from build123d import *

# Parameters (mm, degrees)
SKETCH1_W                        = 92.075
SKETCH1_H                        = 15.875
BOSS_EXTRUDE1_DEPTH              = 15.875
SKETCH2_W                        = 47.625
SKETCH2_H                        = 15.875
CUT_EXTRUDE1_DEPTH               = 52.219943931
F_10_0_1935_DIAMETER_HOLE1_D     = 5.1054
F_10_START                       = -7.9375
F_10_0_1935_DIAMETER_SLOT1_DEPTH = 15.875
CUT_EXTRUDE2_REACH               = 51.34
SKETCH7_W                        = 47.625
SKETCH7_H                        = 12.065
CUT_EXTRUDE3_REACH               = 58.485
SKETCH8_W                        = 38.1
SKETCH8_H                        = 9.525
SKETCH9_W                        = 18.415
SKETCH9_H                        = 15.875
BOSS_EXTRUDE2_DEPTH              = 3.81


# Read off the part's stored shape, not the designer's step: #10 (0.1935) Diameter Slot1
with BuildPart() as part:
    # Sketch1 → Boss-Extrude1 (new, symmetric)
    with BuildSketch(Plane(origin=(0, 0, 0), x_dir=(1, 0, 0), z_dir=(0, 1, 0))):
        Rectangle(SKETCH1_W, SKETCH1_H)
    extrude(amount=BOSS_EXTRUDE1_DEPTH, both=True)

    # Sketch2 → Cut-Extrude1 (cut, through all)
    with BuildSketch(Plane.XY.offset(7.9375)):
        with Locations((-22.225, 7.9375)):
            Rectangle(SKETCH2_W, SKETCH2_H)
    extrude(amount=-CUT_EXTRUDE1_DEPTH, mode=Mode.SUBTRACT)

    # #10 (0.1935) Diameter Hole1 (through all)
    with Locations(Plane.XY.offset(7.9375)):
        with Locations((33.3375, 9.525), (20.6375, 9.525)):
            Hole(F_10_0_1935_DIAMETER_HOLE1_D / 2)

    # #10 (0.1935) Diameter Slot1 outline → #10 (0.1935) Diameter Slot1 (cut)
    with BuildSketch(Plane.XY.offset(F_10_START)):
        with BuildLine():
            ThreePointArc((-23.1902, -10.4902), (-20.6375, -7.9375), (-23.1902, -5.3848))
            Line((-23.1902, -5.3848), (-46.0375, -5.3848))
            Line((-46.0375, -5.3848), (-46.0375, -10.4902))
            Line((-46.0375, -10.4902), (-23.1902, -10.4902))
        make_face()
    extrude(amount=F_10_0_1935_DIAMETER_SLOT1_DEPTH, mode=Mode.SUBTRACT)

    # Sketch7 → Cut-Extrude2 (cut, up to next)
    with BuildSketch(Plane(origin=(0, 0, 0), x_dir=(1, 0, 0), z_dir=(0, 1, 0)), mode=Mode.PRIVATE) as cut_extrude2_sk1:
        with Locations((-22.225, 1.905)):
            Rectangle(SKETCH7_W, SKETCH7_H)
    cut_extrude2_tool1 = extrude(cut_extrude2_sk1.sketch, amount=-CUT_EXTRUDE2_REACH, mode=Mode.PRIVATE) & part.part
    add(cut_extrude2_tool1.solids().sort_by_distance((-22.225, 0, -1.905))[0], mode=Mode.SUBTRACT)

    # Sketch8 → Cut-Extrude3 (cut, up to next)
    with BuildSketch(Plane(origin=(0, 15.875, 0), x_dir=(1, 0, 0), z_dir=(0, 1, 0)), mode=Mode.PRIVATE) as cut_extrude3_sk1:
        with Locations((26.9875, -3.175)):
            Rectangle(SKETCH8_W, SKETCH8_H)
    cut_extrude3_tool1 = extrude(cut_extrude3_sk1.sketch, amount=-CUT_EXTRUDE3_REACH, mode=Mode.PRIVATE) & part.part
    add(cut_extrude3_tool1.solids().sort_by_distance((26.9875, 15.875, 3.175))[0], mode=Mode.SUBTRACT)

    # Sketch9 → Boss-Extrude2 (add)
    with BuildSketch(Plane(origin=(0, 0, 4.1275), x_dir=(-1, 0, 0), z_dir=(0, 0, -1))):
        with Locations((7.62, -7.9375)):
            Rectangle(SKETCH9_W, SKETCH9_H)
    extrude(amount=BOSS_EXTRUDE2_DEPTH)


solid = part.part
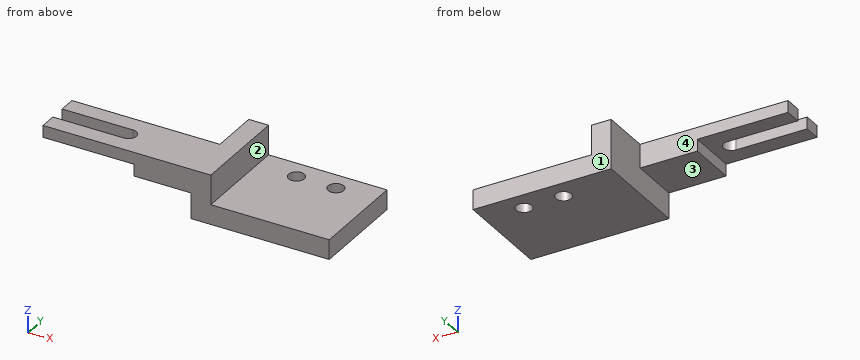
Geometry: final body of the model. Coordinates: model frame, mm. Face numbers are marked on the shaded views. A direction names the side the tool comes from. Round coordinates to 2 decimals unless told otherwise and drop trailing zeros. Loops run counter-clockwise (first coordinate to the right, second up) from the corner with the lowest first, then second, coordinate; pieces in that order, holes last. Notation, with made-up numbers: (64, -26) -> (99, -26) arc R18 ccw to (99, -19) -> close; hole circle Ø11 at (9.25, -30). An arc over 180 degrees is marked (long way). One line per question, with ' | ' between items. Start each with the question number.
1. Set-up query: the marked faces 1, 2, 3 and 4. Return all of +Z, -Z, +X, -X, +Y, -Y with unobstructed straight access to the full face (end or side cutting, diameter ignored); none if empty.
2. Section B-B on x = 32.5. Output: boundary loops of the cut face in (y, z) (1 decimal).
3. Contact query for flat-ended pins moving along their axis: pin 1 (5 mm diameter, centred on y = -0.5, z = -2, fed in from -X); pin 2 (4 mm diameter, centred on x = -38.5, z = 5.5, fed in from +Y); pin 3 (1 mm diameter, centred on y = -8, z = 5.5, fed in from +X); pin 4 (3 mm diameter, centred on x = 20.64, y = 9.52, fed in from -Z). Output: stop coordinate, or through.
4. Section C-C on x = -3. Output: boundary loops of the cut face in (y, z) (1 decimal).
5. Section A-A on y = -3. Output: boundary loops of the cut face in (x, z), and give its area (3 significant figures).
6. Section D-D on z = -2.75. Output: boundary loops of the cut face in (x, y) (1 decimal).
7. Line query: line 1 along X through (y, z) = (9.5, -3); line 2 along Y through (x, z) = (-33.5, 6.5) (3 decimals); line 3 along X through (y, z) = (14, -6). Output: solid intervals per line, ascending. Write a range as [from, to].
Returned:
1) face 1: +Z, -Z, +X, -X, +Y | face 2: +Z, +X, +Y, -Y | face 3: -Z, -X, +Y, -Y | face 4: +Z, -Z, -X, +Y
2) outline: (-15.9, -7.9) -> (7.1, -7.9) -> (7.1, -1.6) -> (-15.9, -1.6) -> close; (11.9, -7.9) -> (15.9, -7.9) -> (15.9, -1.6) -> (11.9, -1.6) -> close
3) pin 1: stops at x = -16.83 | pin 2: stops at y = 0 | pin 3: stops at x = 7.94 | pin 4: passes through
4) outline: (-15.9, 0.3) -> (0, 0.3) -> (0, 7.9) -> (-15.9, 7.9) -> close
5) outline: (-46.04, 4.13) -> (-16.83, 4.13) -> (-16.83, 0.32) -> (1.59, 0.32) -> (1.59, -7.94) -> (46.04, -7.94) -> (46.04, -1.59) -> (7.94, -1.59) -> (7.94, 7.94) -> (-46.04, 7.94) -> close | area: 594 mm2
6) outline: (1.6, -15.9) -> (46, -15.9) -> (46, 15.9) -> (1.6, 15.9) -> close; hole circle Ø5.1 at (20.6, 9.5); hole circle Ø5.1 at (33.3, 9.5)
7) line 1: x = [1.59, 18.08], [23.19, 30.78], [35.89, 46.04] | line 2: y = [-15.875, -10.49], [-5.385, 0] | line 3: x = [1.59, 46.04]
